```python
from build123d import *

# Parameters (mm, degrees)
EXTRUDE_2_DEPTH          = 10
CHAMFER_1_SIZE           = 2
SKETCH_9_R               = 7.5
EXTRUDE_7_DEPTH          = 20
CUT_EXTRUDE_3_DEPTH      = 24
CUT_EXTRUDE_3_DEPTH_BACK = 197.596032513
SKETCH_11_R              = 5
EXTRUDE_8_DEPTH          = 12


with BuildPart() as part:
    # 草图1 → 凸台-拉伸2 (new body)
    with BuildSketch(Plane(origin=(0, 0, 0), x_dir=(1, 0, 0), z_dir=(0, 1, 0))):
        with BuildLine():
            Line((0, 15), (180, 15))
            ThreePointArc((180, 15), (195, 0), (180, -15))
            Line((180, -15), (0, -15))
            ThreePointArc((0, -15), (-15, 0), (0, 15))
        make_face()
    extrude(amount=EXTRUDE_2_DEPTH)

    # 倒角1
    chamfer_1_edges = [part.edges().sort_by_distance(p)[0] for p in [
        (90, 10, -15),
        (-15, 10, 0),
        (90, 10, 15),
        (-15, 0, 0),
        (90, 0, -15),
        (195, 0, 0),
        (90, 0, 15),
        (195, 10, 0),
    ]]
    chamfer(chamfer_1_edges, length=CHAMFER_1_SIZE)

    # 草图9 → 凸台-拉伸7 (add)
    with BuildSketch(Plane.XZ):
        with Locations(Location((0, 0, 0), (0, 0, 90))):
            Circle(SKETCH_9_R)
    extrude(amount=EXTRUDE_7_DEPTH)

    # 草图4 → 切除-拉伸3 (cut, two sides: drawn at the far end of the back side and taken through both)
    with BuildSketch(Plane.XZ.offset(-CUT_EXTRUDE_3_DEPTH_BACK)):
        with BuildLine():
            Line((4, 3), (4, -3))
            ThreePointArc((4, -3), (-5, 0), (4, 3))
        make_face()
    extrude(amount=CUT_EXTRUDE_3_DEPTH + CUT_EXTRUDE_3_DEPTH_BACK, mode=Mode.SUBTRACT)

    # 草图11 → 凸台-拉伸8 (add)
    with BuildSketch(Plane.XZ):
        with Locations(Location((180, 0, 0), (0, 0, 90))):
            Circle(SKETCH_11_R)
    extrude(amount=EXTRUDE_8_DEPTH)


solid = part.part
```
Build history of the part. All positions in model axes, mm. A direction names the side the tool comes from. Round coordinates to 2 decimals unless told otherwise and drop trailing zeros. Write each loop counter-clockwise with the first axis right and the second up, starting at its lowest first coordinate (ties: lowest second). Pieces come first, ordered by that corner, then holes. Notation, with made-up numbers: (12, 5.25) - (20, 5.25) arc R12 cw to (20, 10.25) - close; hole circle Ø10 at (52.25, 76.5). An arc over 180 degrees is marked (long way). Answer as CSV lines item,"result".
Q1. Cut at C-C (z = 0). Write the cut outline in (x, y), and give its area (3 significant figures).
Report:
outline,"(-15, 2) - (-13, 0) - (-7.5, 0) - (-7.5, -20) - (-5, -20) - (-5, 10) - (-13, 10) - (-15, 8) - close; (4, -20) - (7.5, -20) - (7.5, 0) - (175, 0) - (175, -12) - (185, -12) - (185, 0) - (193, 0) - (195, 2) - (195, 8) - (193, 10) - (4, 10) - close"
area,"2,240 mm^2"
Q2. Drill centre lines: probe 1 along X at (y, z) = (-5.5, 0); probe 2 along X at (y, z) = (-17.5, 0); probe 3 along Z at (x, y) = (0, 2.25). Where is each one in solid material? Low to high. Write a range as [from, to].
Report:
probe 1,"x = [-7.5, -5], [4, 7.5], [175, 185]"
probe 2,"x = [-7.5, -5], [4, 7.5]"
probe 3,"z = [-15, -5], [5, 15]"
Q3. Cut at A-A (y = -6). Write the cut outline in (x, z), and give its area (3 significant figures).
Report:
outline,"circle Ø15 at (0, 0); circle Ø10 at (180, 0); hole (4, -3) - (4, 3) arc R5 ccw (long way) to start"
area,"181 mm^2"
Q4. Drop flat-ended pins along their axis: pin 1 (8 mm diameter, centred on x = 139.5, z = -2.5, fed in from -Y); pin 2 (8 mm diameter, centred on x = 180, z = 0.5, fed in from -Y); pin 3 (6.5 mm diameter, centred on y = 1, z = 1, fed in from -X); pin 4 (6 mm diameter, centred on y = -8.5, z = 6.5, fed in from +X). Give the stop position or say it passes through.
Report:
pin 1,"stops at y = 0"
pin 2,"stops at y = -12"
pin 3,"stops at x = -15"
pin 4,"stops at x = 183.57"
Q5. Cut at B-B (x = 107.5). Write the cut outline in (y, z), and give its area (3 significant figures).
Report:
outline,"(0, -13) - (2, -15) - (8, -15) - (10, -13) - (10, 13) - (8, 15) - (2, 15) - (0, 13) - close"
area,"292 mm^2"
Q6. Tool access for faces 4 (the cylindrical face through (175.043, -5.916, -0.651)), 5 (the flat face through (4, -5, 0)), 6 (the flat face through (180, -12, 0)): list every direction of +Z, -Z, +X, -X, +Y, -Y with a clear straight run to the whole face (end or side of a thin tool).
Report:
face 4,"-Y"
face 5,"+Y, -Y"
face 6,"+Z, -Z, +X, -Y"
Q7. Cut at D-D (y = -15). Write the cut outline in (x, z).
Report:
outline,"circle Ø15 at (0, 0); hole (4, -3) - (4, 3) arc R5 ccw (long way) to start"
Q8. Pull direction Z, two halves, no side cores. Call faces 1 (the cylindrical face through (-0.33, -9.86, -7.493)), 2 (the flat face through (89, 5, -15)), 3 (the cylindrical face through (-5, -5, 0)): +Z half, -Z half, draft (parallel to the pull), parting line (faces both ways), or undercut.
Report:
face 1,"parting line"
face 2,"-Z half"
face 3,"undercut"
